Part print with two shaded views. Sizes in mm from the minimum x, y, z corner. A direction names the side the tool comes from. Give positions to 0.01 mm unless a question says otherwise; leave off trailing zeros. Order: outer loops, then holes, each group sorted by start corner. A loop starts at its lowest first (then second) coordinate and runs counter-clockwise, first axis right, second up. Notation, with made-up numbers: (-17, 5.25) - (21, 5.25) arc R17 ccw to (21, 9.25) - close; hole circle Ø11 at (73.25, 40). An arc over 180 degrees is marked (long way). Return JSON: item names as keys, results as strings. Group by question number.
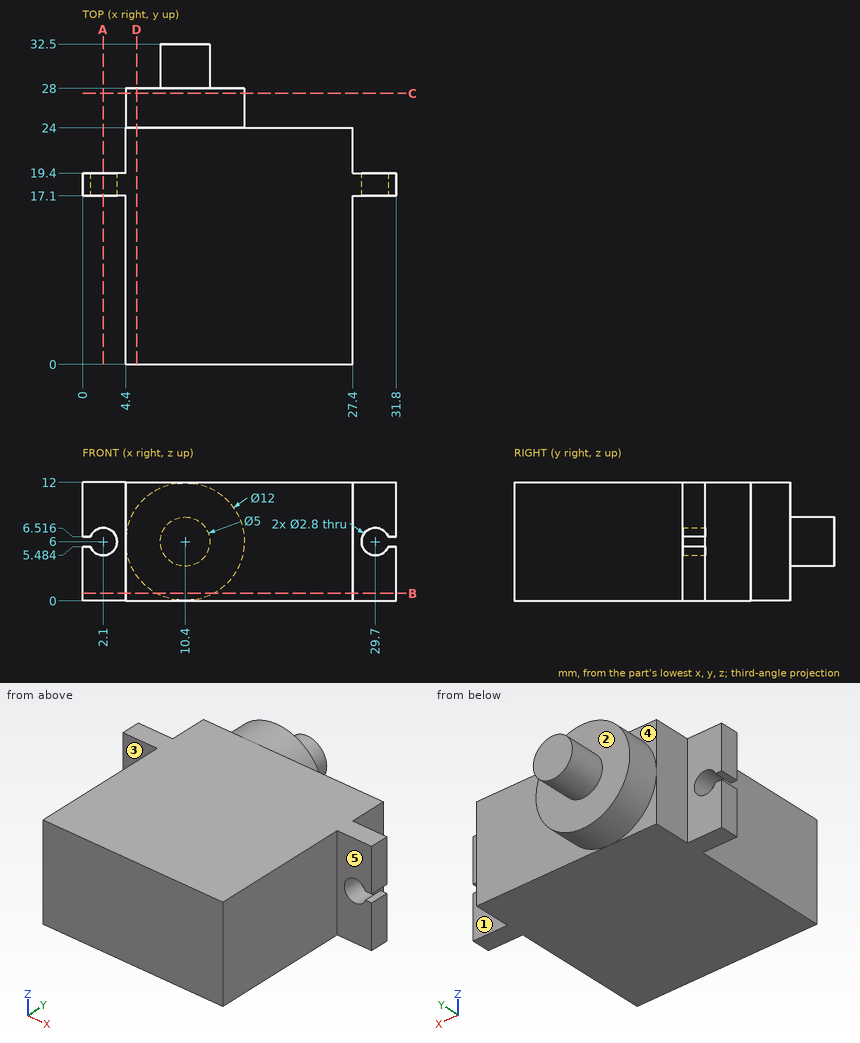
(1) Slice it at A-A (x = 2.1). Give the cut face in (y, z).
(2) Drop flat-ended pins along their axis: pin 1 Ø3 at (y, z) = (14.5, 4.5) entering from -X; pin 2 Ø2 at (x, z) = (28.5, 8.5) entering from +Y; pin 3 Ø2 at (x, z) = (24.5, 1.5) entering from +Y. Give the stop position or say it passes through.
(3) Slice it at D-D (x = 5.5). Give the cut face in (y, z), and give its area (3 significant figures).
(4) Slice it at C-C (y = 27.5). Give the cut face in (x, z).
(5) Drill centre lines: L1, parallel to Z at x = 29.7, y = 17.8; L2, parallel to Y at x = 17, z = 6; L3, parallel to X at y = 10, z = 11.5. Where is each one in solid material? Low to high.
(6) 3-axis set-ups, long thin cutter, end or side, ignore diameter. For the marked faces 1, 2, 3, 4 and 5: which of +Z, -Z, +X, -X, +Y, -Y reach the whole face in a straight line?
(7) Slice it at B-B (z = 0.75). Give the cut face in (x, y) (1 decimal).
Result set:
{
 "1": {"outline": "(17.1, 0) - (19.4, 0) - (19.4, 4.6) - (17.1, 4.6) - close; (17.1, 7.4) - (19.4, 7.4) - (19.4, 12) - (17.1, 12) - close"},
 "2": {"pin 1": "stops at x = 4.4", "pin 2": "stops at y = 19.4", "pin 3": "stops at y = 24"},
 "3": {"outline": "(0, 0) - (24, 0) - (24, 2.54) - (28, 2.54) - (28, 9.46) - (24, 9.46) - (24, 12) - (0, 12) - close", "area": "316 mm²"},
 "4": {"outline": "circle Ø12 at (10.4, 6)"},
 "5": {"L1": "z = 0 to 4.6, 7.4 to 12", "L2": "y = 0 to 24", "L3": "x = 4.4 to 27.4"},
 "6": {"face 1": "+Z, -Z, +X, +Y", "face 2": "+Y", "face 3": "+Z, -Z, -X, -Y", "face 4": "+Z, -X, +Y", "face 5": "+Z, -Z, +X, -Y"},
 "7": {"outline": "(0, 17.1) - (4.4, 17.1) - (4.4, 0) - (27.4, 0) - (27.4, 17.1) - (31.8, 17.1) - (31.8, 19.4) - (27.4, 19.4) - (27.4, 24) - (13.3, 24) - (13.3, 28) - (7.5, 28) - (7.5, 24) - (4.4, 24) - (4.4, 19.4) - (0, 19.4) - close"}
}
